Here's how the part is built. I have some questions about the finished solid (model axes, mm). Face numbers are marked on the shaded views. Round coordinates to 2 decimals unless told otherwise and drop trailing zeros. Write each loop counter-clockwise with the first axis right and the second up, starting at its lowest first coordinate (ties: lowest second). Pieces come first, ordered by that corner, then holes. Notation, with made-up numbers: (69, 57.25) -> (73, 57.25) arc R26 cw to (73, 80.25) -> close; hole circle Ø1 at (62.25, -4). An arc over 180 degrees is marked (long way). Put each result on its own line as item: value. Start each with the question number.
1. Suppose I cut it at B-B (z = -6.25). Please give me the cut outline in (x, y).
2. I need wall thicknesses on probe 1 along Y at (x, z) = (28, -3.25); probe 2 along Y at (x, z) = (29, -4); probe 3 along X at (y, z) = (18, -1.75). Which ranges of each line are inside material? Lowest first, please. Write a range as from..to.
3. Suppose I cut it at D-D (y = -21). Please give me the cut outline in (x, z), then the cut area to 3 significant figures.
4. We'd pull the mould along Y, two halves only. Please class the marked faces 1, 2, 3 and 4: +Y half, -Y half, draft (parallel to the pull), parting line (faces both ways), or undercut.
5. Suppose I cut it at A-A (y = 32). Please give me the cut outline in (x, z), then the cut area to 3 significant figures.
6. For pin 1 (9.5 mm diameter, centred on x = -92, y = 32, fed in from +Z); pin 2 (5 mm diameter, centred on y = -2.5, z = -5, fed in from +X); pin 3 (2 mm diameter, centred on y = -13.5, z = -4, fed in from +X); pin 4 (2 mm diameter, centred on y = -7, z = 1.5, fed in from +X), each with a flat end and sliding along its axis, tell me the tip position at first contact or that it passes through.
7. Suppose I cut it at C-C (x = -92). Please give me the cut outline in (y, z), then the cut area to 3 significant figures.
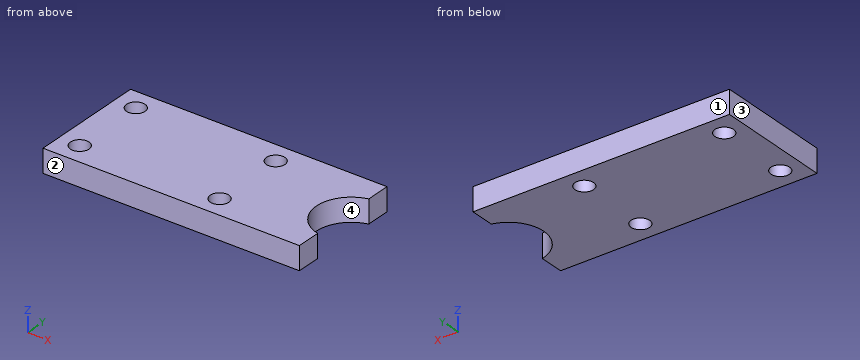
```python
from build123d import *

# Parameters (mm, degrees)
F0_R     = 8
F1_DEPTH = 10


with BuildPart() as f1:
    # F0 (on Top) → F1 (new body, symmetric)
    with BuildSketch(Plane.XY):
        with BuildLine():
            Line((-110, -50), (110, -50))
            Line((110, -50), (110, -29.171904))
            ThreePointArc((110, -29.171904), (87, 0), (110, 29.171904))
            Line((110, 29.171904), (110, 50))
            Line((110, 50), (-110, 50))
            Line((-110, 50), (-110, -50))
        make_face()
        with Locations((-92, -32)):
            Circle(F0_R, mode=Mode.SUBTRACT)
        with Locations((28, -32)):
            Circle(F0_R, mode=Mode.SUBTRACT)
        with Locations((-92, 32)):
            Circle(F0_R, mode=Mode.SUBTRACT)
        with Locations((28, 32)):
            Circle(F0_R, mode=Mode.SUBTRACT)
    extrude(amount=F1_DEPTH, both=True)


solid = f1.part
```
Verdict:
1. outline: (-110, -50) -> (110, -50) -> (110, -29.17) arc R30 cw to (110, 29.17) -> (110, 50) -> (-110, 50) -> close; hole circle Ø16 at (-92, -32); hole circle Ø16 at (-92, 32); hole circle Ø16 at (28, -32); hole circle Ø16 at (28, 32)
2. probe 1: y = -50..-40, -24..24, 40..50
2. probe 2: y = -50..-39.94, -24.06..24.06, 39.94..50
2. probe 3: x = -110..93
3. outline: (-110, -10) -> (95.58, -10) -> (95.58, 10) -> (-110, 10) -> close
3. area: 4,110 mm^2
4. face 1: +Y half
4. face 2: -Y half
4. face 3: draft
4. face 4: undercut
5. outline: (-110, -10) -> (-100, -10) -> (-100, 10) -> (-110, 10) -> close; (-84, -10) -> (20, -10) -> (20, 10) -> (-84, 10) -> close; (36, -10) -> (110, -10) -> (110, 10) -> (36, 10) -> close
5. area: 3,760 mm^2
6. pin 1: passes through
6. pin 2: stops at x = 87.42
6. pin 3: stops at x = 90.74
6. pin 4: stops at x = 88.09
7. outline: (-50, -10) -> (-40, -10) -> (-40, 10) -> (-50, 10) -> close; (-24, -10) -> (24, -10) -> (24, 10) -> (-24, 10) -> close; (40, -10) -> (50, -10) -> (50, 10) -> (40, 10) -> close
7. area: 1,360 mm^2
